Can you work these out from the drawing? Everything is in mm from the part's minimum corner. A direction names the side the tool comes from. Round coordinates to 2 decimals unless told otherwise and drop trailing zeros. Order: outer loops, then holes, each group sorted by start corner. A loop starts at its lowest first (then second) coordinate and runs counter-clockwise, first axis right, second up. Notation, with made-up numbers: (78.25, 8) -> (86.25, 8) arc R22 cw to (86.25, 17) -> close; hole circle Ø11 at (-40, 35.5). An arc over 180 degrees is marked (long way). One line per item, written item: value.
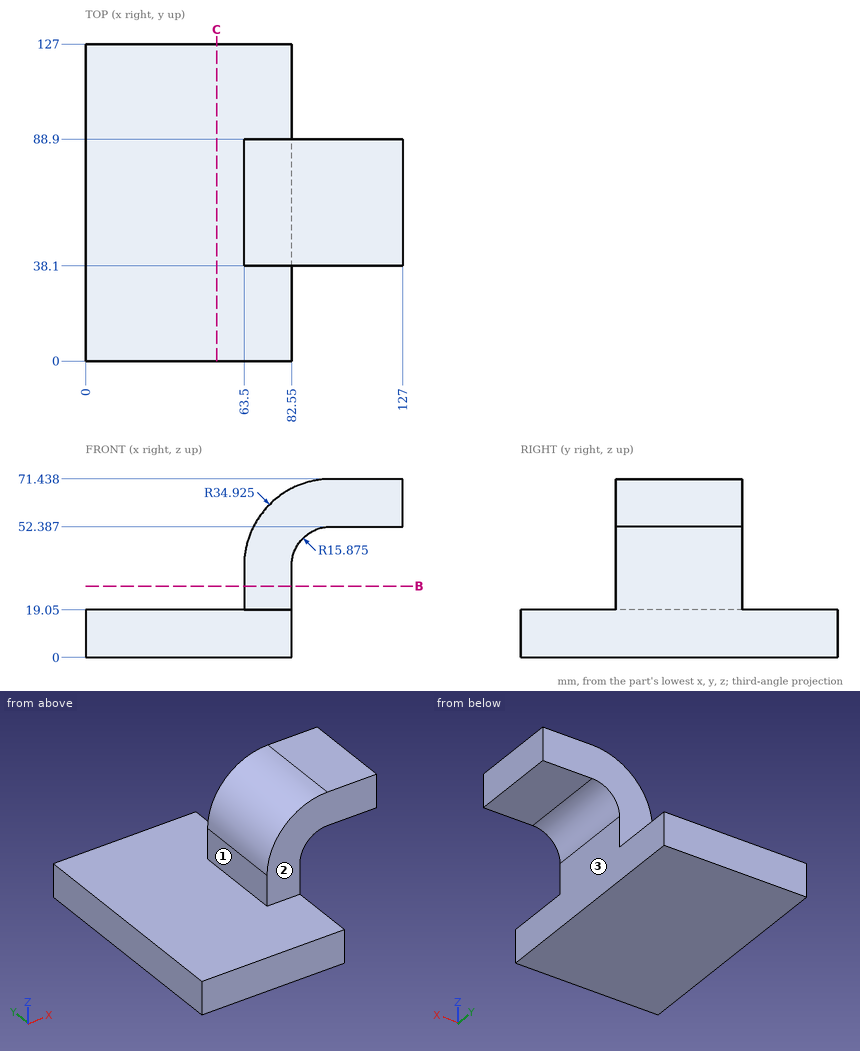
Q1. I want a section at B-B on z = 28.5. Write out the boundary of the cut face in (x, y), then the cut area to 3 significant figures.
Answers:
outline: (63.5, 38.1) -> (82.55, 38.1) -> (82.55, 88.9) -> (63.5, 88.9) -> close
area: 968 mm2
Q2. For P1, Ø18.5, axis at y = 39.5, z = 12.5, coming from the +X side; P2, Ø2, axis at y = 69.5, z = 46.5, coming from the +X side (1 decimal); P3, Ø8.5, axis at y = 74, z = 24, coming from the -X side; P4, Ø15.5, axis at x = 109.5, z = 41, coming from the +Y side (3 decimals), each with a flat end and sliding along its axis, tell me the tip position at first contact or that it passes through.
Answers:
P1: x = 82.55
P2: x = 87
P3: x = 63.5
P4: through
Q3. I want a section at C-C on x = 52.5. Write out the boundary of the cut face in (y, z), then the cut area to 3 significant figures.
Answers:
outline: (0, 0) -> (127, 0) -> (127, 19.05) -> (0, 19.05) -> close
area: 2,420 mm2
Q4. I need wall thicknesses on line 1 along Z through (x, y) = (10, 91.5); line 2 along Z through (x, y) = (99.5, 85); line 3 along X through (y, z) = (58, 35). Which ranges of each line are inside material? Lowest first, please.
Answers:
line 1: 0 to 19.05
line 2: 52.39 to 71.44
line 3: 63.5 to 82.55
Q5. Which directions (+Z, -Z, +X, -X, +Y, -Y) give clear straight access to the entire face, cutting with the end or side of a thin tool? Please do the marked faces 1, 2 and 3.
Answers:
face 1: +Z, -X, +Y, -Y
face 2: +Z, +X, -X, -Y
face 3: -Z, +X, +Y, -Y
